Work out the finished part from the listing and answer in its coordinate system (mm). A direction names the side the tool comes from. Coordinates: 2 decimals unless noted, no trailing zeros. Order: outer loops, then holes, each group sorted by start corner. A loop starts at its lowest first (then second) coordinate and runs counter-clockwise, first axis right, second up. Notation, with made-up numbers: (-24.5, 10) -> (25.5, 10) arc R23 cw to (25.5, 32) -> close; hole circle Ø6 at (59, 87.5). An arc over 180 degrees is marked (long way). Use one line per item in the form item = value.
from build123d import *

# Parameters (mm, degrees)
SKETCH_1_R               = 20
EXTRUDE_1_DEPTH          = 15
SKETCH_2_R               = 2.5
CUT_EXTRUDE_1_DEPTH      = 5
MIRROR_2_COPY_1_SKETCH_R = 2.5
MIRROR_2_COPY_1_DEPTH    = 5
MIRROR_3_COPY_1_SKETCH_R = 2.5
MIRROR_3_COPY_1_DEPTH    = 5
MIRROR_3_COPY_2_SKETCH_R = 2.5
MIRROR_3_COPY_2_DEPTH    = 5
MIRROR_3_COPY_3_SKETCH_R = 2.5
MIRROR_3_COPY_3_DEPTH    = 5


with BuildPart() as part:
    # 草图1 → 凸台-拉伸1 (new body)
    with BuildSketch(Plane(origin=(0, 0, 0), x_dir=(1, 0, 0), z_dir=(0, 1, 0))):
        with BuildLine():
            Line((44.458501576, 15.246036783), (65.781966365, 25.910071498))
            ThreePointArc((65.781966365, 25.910071498), (68.576327064, 34.295567803), (60.190830759, 37.089928502))
            Line((60.190830759, 37.089928502), (38.867365971, 26.425893787))
            ThreePointArc((38.867365971, 26.425893787), (0, 47), (-38.867365971, 26.425893787))
            Line((-38.867365971, 26.425893787), (-60.190830759, 37.089928502))
            ThreePointArc((-60.190830759, 37.089928502), (-68.576327064, 34.295567803), (-65.781966365, 25.910071498))
            Line((-65.781966365, 25.910071498), (-44.458501576, 15.246036783))
            ThreePointArc((-44.458501576, 15.246036783), (-47, 0), (-44.458501576, -15.246036783))
            Line((-44.458501576, -15.246036783), (-65.781966365, -25.910071498))
            ThreePointArc((-65.781966365, -25.910071498), (-68.576327064, -34.295567803), (-60.190830759, -37.089928502))
            Line((-60.190830759, -37.089928502), (-38.867365971, -26.425893787))
            ThreePointArc((-38.867365971, -26.425893787), (0, -47), (38.867365971, -26.425893787))
            Line((38.867365971, -26.425893787), (60.190830759, -37.089928502))
            ThreePointArc((60.190830759, -37.089928502), (68.576327064, -34.295567803), (65.781966365, -25.910071498))
            Line((65.781966365, -25.910071498), (44.458501576, -15.246036783))
            ThreePointArc((44.458501576, -15.246036783), (47, 0), (44.458501576, 15.246036783))
        make_face()
        with Locations(Location((0, 0, 0), (0, 0, 270))):
            Circle(SKETCH_1_R, mode=Mode.SUBTRACT)
    extrude(amount=EXTRUDE_1_DEPTH)

    # 草图2 → 切除-拉伸1 (cut)
    with BuildSketch(Plane(origin=(0, 15, 0), x_dir=(1, 0, 0), z_dir=(0, 1, 0))):
        with Locations(Location((-62.986398562, 31.5, 0), (0, 0, 270))):
            Circle(SKETCH_2_R)
    cut_extrude_1 = extrude(amount=-CUT_EXTRUDE_1_DEPTH, mode=Mode.SUBTRACT)

    # 镜向1: 切除-拉伸1 across plane
    add(cut_extrude_1.mirror(Plane.XY), mode=Mode.SUBTRACT)

    # 镜向2: 切除-拉伸1 across plane
    add(cut_extrude_1.mirror(Plane(origin=(0, 0, 0), x_dir=(0, 0, 1), z_dir=(1, 0, 0))), mode=Mode.SUBTRACT)

    # 镜向2 copy 1 sketch → 镜向2 copy 1 (cut)
    with BuildSketch(Plane(origin=(0, 15, 0), x_dir=(-1, 0, 0), z_dir=(0, 1, 0))):
        with Locations(Location((-62.986398562, 31.5, 0), (0, 0, 270))):
            Circle(MIRROR_2_COPY_1_SKETCH_R)
    extrude(amount=-MIRROR_2_COPY_1_DEPTH, mode=Mode.SUBTRACT)

    # 镜向3: 切除-拉伸1 across plane
    add(cut_extrude_1.mirror(Plane(origin=(0, 7.5, 0), x_dir=(0, 0, 1), z_dir=(0, -1, 0))), mode=Mode.SUBTRACT)

    # 镜向3 copy 1 sketch → 镜向3 copy 1 (cut)
    with BuildSketch(Plane.XZ):
        with Locations(Location((-62.986398562, 31.5, 0), (0, 0, 270))):
            Circle(MIRROR_3_COPY_1_SKETCH_R)
    extrude(amount=-MIRROR_3_COPY_1_DEPTH, mode=Mode.SUBTRACT)

    # 镜向3 copy 2 sketch → 镜向3 copy 2 (cut)
    with BuildSketch(Plane(origin=(0, 0, 0), x_dir=(-1, 0, 0), z_dir=(0, -1, 0))):
        with Locations(Location((-62.986398562, 31.5, 0), (0, 0, 270))):
            Circle(MIRROR_3_COPY_2_SKETCH_R)
    extrude(amount=-MIRROR_3_COPY_2_DEPTH, mode=Mode.SUBTRACT)

    # 镜向3 copy 3 sketch → 镜向3 copy 3 (cut)
    with BuildSketch(Plane(origin=(0, 0, 0), x_dir=(-1, 0, 0), z_dir=(0, -1, 0))):
        with Locations((-62.986398562, -31.5)):
            Circle(MIRROR_3_COPY_3_SKETCH_R)
    extrude(amount=-MIRROR_3_COPY_3_DEPTH, mode=Mode.SUBTRACT)


solid = part.part
(1) Section D-D on y = 3.5 is taken. Write down the section's boundary in (x, z).
Data:
outline = (-65.78, -25.91) arc R6.25 ccw to (-60.19, -37.09) -> (-38.87, -26.43) arc R47 ccw to (38.87, -26.43) -> (60.19, -37.09) arc R6.25 ccw to (65.78, -25.91) -> (44.46, -15.25) arc R47 ccw to (44.46, 15.25) -> (65.78, 25.91) arc R6.25 ccw to (60.19, 37.09) -> (38.87, 26.43) arc R47 ccw to (-38.87, 26.43) -> (-60.19, 37.09) arc R6.25 ccw to (-65.78, 25.91) -> (-44.46, 15.25) arc R47 ccw to (-44.46, -15.25) -> close; hole circle Ø5 at (-62.99, -31.5); hole circle Ø5 at (-62.99, 31.5); hole circle Ø40 at (0, 0); hole circle Ø5 at (62.99, -31.5); hole circle Ø5 at (62.99, 31.5)
(2) Section C-C on z = 31.5 is taken. Write down the section's boundary in (x, y), plus the area to 3 significant figures.
Data:
outline = (-69.24, 0) -> (-65.49, 0) -> (-65.49, 5) -> (-60.49, 5) -> (-60.49, 0) -> (-49.01, 0) -> (-49.01, 15) -> (-60.49, 15) -> (-60.49, 10) -> (-65.49, 10) -> (-65.49, 15) -> (-69.24, 15) -> close; (-34.88, 0) -> (34.88, 0) -> (34.88, 15) -> (-34.88, 15) -> close; (49.01, 0) -> (60.49, 0) -> (60.49, 5) -> (65.49, 5) -> (65.49, 0) -> (69.24, 0) -> (69.24, 15) -> (65.49, 15) -> (65.49, 10) -> (60.49, 10) -> (60.49, 15) -> (49.01, 15) -> close
area = 1,550 mm²
(3) Which of the six approach directions +Z, -Z, +X, -X, +Y, -Y give full straight-line access (tool end or side, diameter ignored) to faces 1 (the flat face through (-63, 5, 32)), 2 (the flat face through (54.971, 7.395, -20.503)), 3 (the flat face through (-63, 10, 32)), 4 (the flat face through (-49.38, 7.395, -31.683)), 5 (the flat face through (-49.678, 7.395, 31.833))?
Data:
face_1 = -Y
face_2 = +X, +Y, -Y
face_3 = +Y
face_4 = -Z, +Y, -Y
face_5 = +Z, +Y, -Y
(4) Straight lines are drawn through the part: line 1 along X through (y, z) = (12.1, -31.5); line 2 along X through (y, z) = (2, -31); line 3 along X through (y, z) = (2, 26.5). For each, find the intervals that lie inside material, in ascending order.
Data:
line_1 = -69.24 to -65.49, -60.49 to -49.01, -34.88 to 34.88, 49.01 to 60.49, 65.49 to 69.24
line_2 = -69.22 to -65.44, -60.54 to -48.01, -35.33 to 35.33, 48.01 to 60.54, 65.44 to 69.22
line_3 = -66.74 to -39.02, -38.82 to 38.82, 39.02 to 66.74
(5) Section B-B on x = 0 is taken. Write down the section's boundary in (y, z).
Data:
outline = (0, -47) -> (15, -47) -> (15, -20) -> (0, -20) -> close; (0, 20) -> (15, 20) -> (15, 47) -> (0, 47) -> close
(6) The mould has two halves that part along X. Classify faces 6 (the flat face through (-54.971, 7.395, 20.503)), 7 (the flat face through (-1, 0, 20.2)), 8 (the cylindrical face through (47, 7, 0)), 9 (the flat face through (63, 10, 32)): released by +X, released by -X, zero draft, split by the parting line, or undercut.
Data:
face_6 = released by -X
face_7 = zero draft
face_8 = released by +X
face_9 = undercut
(7) Each of these flat-tipped pins is pushed along its axis until it touches: P1, Ø6, axis at y = 13, z = 24.5, coming from the +X side; P2, Ø4, axis at x = -63, z = 31.5, coming from the +Y side; P3, Ø6, axis at x = 32, y = 6.5, coming from the -Z side; P4, Ø1.5, axis at x = 47.5, z = -33.5, coming from the -Y side (3 decimals). Where does it stop, or does it pass through?
Data:
P1 = 67.79
P2 = 10
P3 = -36.99
P4 = through
(8) Section A-A on z = 0 is taken. Write down the section's boundary in (x, y), plus the area to 3 significant figures.
Data:
outline = (-47, 0) -> (-20, 0) -> (-20, 15) -> (-47, 15) -> close; (20, 0) -> (47, 0) -> (47, 15) -> (20, 15) -> close
area = 810 mm²
